from build123d import *

# Parameters (mm, degrees)
F0_W     = 20
F0_H     = 20
F1_DEPTH = 20
F2_R     = 2.6
F3_DEPTH = 1
F4_R     = 2.6
F5_DEPTH = 1
F6_R     = 2.6
F7_DEPTH = 1


with BuildPart() as f1:
    # F0 (on Front) → F1 (new body)
    with BuildSketch(Plane.XZ):
        with Locations((10, 10)):
            Rectangle(F0_W, F0_H)
    extrude(amount=F1_DEPTH)

    # F2 (on face) → F3 (cut)
    with BuildSketch(Plane(origin=(0, 0, 0), x_dir=(0, -1, 0), z_dir=(-1, 0, 0))):
        with Locations((10, 10)):
            Circle(F2_R)
        with Locations((5, 15)):
            Circle(F2_R)
        with Locations((15, 15)):
            Circle(F2_R)
        with Locations((15, 5)):
            Circle(F2_R)
        with Locations((5, 5)):
            Circle(F2_R)
    extrude(amount=-F3_DEPTH, mode=Mode.SUBTRACT)

    # F4 (on face) → F5 (cut)
    with BuildSketch(Plane.YZ.offset(20)):
        with Locations((-15, 15)):
            Circle(F4_R)
        with Locations((-5, 5)):
            Circle(F4_R)
    extrude(amount=-F5_DEPTH, mode=Mode.SUBTRACT)

    # F6 (on face) → F7 (cut)
    with BuildSketch(Plane(origin=(0, 0, 0), x_dir=(-1, 0, 0), z_dir=(0, 1, 0))):
        with Locations((-10, 10)):
            Circle(F6_R)
        with Locations((-5, 15)):
            Circle(F6_R)
        with Locations((-15, 5)):
            Circle(F6_R)
    extrude(amount=-F7_DEPTH, mode=Mode.SUBTRACT)


solid = f1.part
CAD build for the part. Positions are in the model's coordinates, mm. A direction names the side the tool comes from. Give positions to 0.01 mm unless a question says otherwise; leave off trailing zeros. Loops run counter-clockwise (first coordinate to the right, second up) from the corner with the lowest first, then second, coordinate; pieces in that order, holes last. Notation, with made-up numbers: M -28.75,73 L 25.25,73 A27 ccw 25.25,99 Z; hole C 24.25,-7 d5. An arc over 180 degrees is marked long. Answer in a Markdown table with one row per item. Add a question column.
Item 1: Band-saw the part on C-C on z = 10. Give the cut face in (x, y), then the cut area to 3 significant figures.
Item 2: Probe probe 1 along Z at (x, y) = (0.3, -5); probe 2 along Z at (x, y) = (5, -0.65); probe 3 along Z at (x, y) = (10, -0.5). List the from-to ranges inside material, lowest first.
Item 3: Tool access for faces 4 (the face through (0.49, -17.48, 5.78)), 5 (the face through (12, 0, 12)), 6 (the face through (19, -15, 15)), 7 (the face through (3.8, -0.493, 12.693)): list every direction of +Z, -Z, +X, -X, +Y, -Y with a clear straight run to the whole face (end or side of a thin tool).
Item 4: Band-saw the part on D-D on y = -16.5. Give the cut face in (x, z).
Item 5: Drop flat-ended pins along their axis: P1, Ø4, axis at x = 10, z = 10, coming from the +Y side; P2, Ø4, axis at y = -5, z = 5, coming from the -X side; P3, Ø2.5, axis at y = -5.5, z = 5.5, coming from the +X side. Give the stop position or say it passes through.
Item 6: Band-saw the part on B-B on y = -6. Give the cut face in (x, z).
Item 7: Mould opens along X. For faces 1 (the face through (10, -10, 20)), 2 (the face through (0, -8, 12)), 3 (the face through (12.52, -0.49, 5.78)) say: +X half, -X half, draft (parallel to the pull), parting line (faces both ways), or undercut.
Item 8: Band-saw the part on A-A on z = 15. Give the cut face in (x, y).
Reply:
| question | item | result |
|---|---|---|
| 1 | outline | M 0,-20 L 20,-20 L 20,0 L 12.6,0 L 12.6,-1 L 7.4,-1 L 7.4,0 L 0,0 L 0,-7.4 L 1,-7.4 L 1,-12.6 L 0,-12.6 Z |
| 1 | area | 390 mm^2 |
| 2 | probe 1 | z = 0 to 2.4, 7.6 to 12.4, 17.6 to 20 |
| 2 | probe 2 | z = 0 to 12.4, 17.6 to 20 |
| 2 | probe 3 | z = 0 to 7.4, 12.6 to 20 |
| 3 | face 4 | -X |
| 3 | face 5 | +Z, -Z, +X, -X, +Y |
| 3 | face 6 | +X |
| 3 | face 7 | +Y |
| 4 | outline | M 0,0 L 20,0 L 20,12.88 L 19,12.88 L 19,17.12 L 20,17.12 L 20,20 L 0,20 L 0,17.12 L 1,17.12 L 1,12.88 L 0,12.88 L 0,7.12 L 1,7.12 L 1,2.88 L 0,2.88 Z |
| 5 | P1 | stops at y = -1 |
| 5 | P2 | stops at x = 1 |
| 5 | P3 | stops at x = 19 |
| 6 | outline | M 0,0 L 20,0 L 20,2.6 L 19,2.6 L 19,7.4 L 20,7.4 L 20,20 L 0,20 L 0,17.4 L 1,17.4 L 1,12.6 L 0,12.6 L 0,7.4 L 1,7.4 L 1,2.6 L 0,2.6 Z |
| 7 | face 1 | draft |
| 7 | face 2 | -X half |
| 7 | face 3 | undercut |
| 8 | outline | M 0,-20 L 20,-20 L 20,-17.6 L 19,-17.6 L 19,-12.4 L 20,-12.4 L 20,0 L 7.6,0 L 7.6,-1 L 2.4,-1 L 2.4,0 L 0,0 L 0,-2.4 L 1,-2.4 L 1,-7.6 L 0,-7.6 L 0,-12.4 L 1,-12.4 L 1,-17.6 L 0,-17.6 Z |
